```python
from build123d import *

# Parameters (mm, degrees)
BOSS_EXTRUDE1_DEPTH = 1.524


with BuildPart() as part:
    # Sketch1 → Boss-Extrude1 (new body)
    with BuildSketch(Plane.XY):
        with BuildLine():
            Line((70.351759676, -1.540442282), (70.351759676, 0))
            Line((70.351759676, 0), (64.929759758, 0))
            ThreePointArc((64.929759758, 0), (64.792973258, 0.011875), (64.660279583, 0.047144684))
            ThreePointArc((64.660279583, 0.047144684), (62.28963908, 2.412826115), (62.588919113, 5.748514423))
            ThreePointArc((62.588919113, 5.748514423), (62.67763825, 5.871916038), (62.788250891, 5.976146011))
            ThreePointArc((62.788250891, 5.976146011), (63.205809067, 6.291372891), (63.63152168, 6.595497187))
            Line((63.63152168, 6.595497187), (65.410554861, 4.41654898))
            Line((65.410554861, 4.41654898), (66.591058918, 5.380388267))
            Line((66.591058918, 5.380388267), (64.92449722, 7.421582138))
            ThreePointArc((64.92449722, 7.421582138), (67.556403706, 8.712737588), (70.349637054, 9.602603653))
            Line((70.349637054, 9.602603653), (70.349637054, 5.958967549))
            Line((70.349637054, 5.958967549), (71.873637054, 5.958967549))
            Line((71.873637054, 5.958967549), (71.873637054, 7.844356511))
            ThreePointArc((71.873637054, 7.844356511), (72.72464753, 6.890883011), (73.797539642, 6.196452982))
            ThreePointArc((73.797539642, 6.196452982), (77.23855889, 3.495988283), (80.283555852, 0.355746802))
            ThreePointArc((80.283555852, 0.355746802), (80.451041219, 0.021581778), (80.447017019, -0.35218475))
            ThreePointArc((80.447017019, -0.35218475), (80.395843158, -0.762), (80.447017019, -1.17181525))
            ThreePointArc((80.447017019, -1.17181525), (80.451041219, -1.545581778), (80.283555852, -1.879746802))
            ThreePointArc((80.283555852, -1.879746802), (77.23855889, -5.019988283), (73.797539642, -7.720452982))
            ThreePointArc((73.797539642, -7.720452982), (72.72464753, -8.414883011), (71.873637054, -9.368356511))
            Line((71.873637054, -9.368356511), (71.873637054, -7.482967549))
            Line((71.873637054, -7.482967549), (70.349637054, -7.482967549))
            Line((70.349637054, -7.482967549), (70.349637054, -11.126603653))
            ThreePointArc((70.349637054, -11.126603653), (67.556403706, -10.236737588), (64.92449722, -8.945582138))
            Line((64.92449722, -8.945582138), (66.591058918, -6.904388267))
            Line((66.591058918, -6.904388267), (65.410554861, -5.94054898))
            Line((65.410554861, -5.94054898), (63.63152168, -8.119497187))
            ThreePointArc((63.63152168, -8.119497187), (63.205809068, -7.815372891), (62.788250891, -7.500146011))
            ThreePointArc((62.788250891, -7.500146011), (62.67763825, -7.395916038), (62.588919113, -7.272514424))
            ThreePointArc((62.588919113, -7.272514424), (62.262802552, -4.01311856), (64.509301597, -1.629160622))
            ThreePointArc((64.509301597, -1.629160622), (64.654260243, -1.585608721), (64.804850415, -1.570364804))
            Line((64.804850415, -1.570364804), (70.351759676, -1.540442282))
        make_face()
    extrude(amount=BOSS_EXTRUDE1_DEPTH)


solid = part.part
```
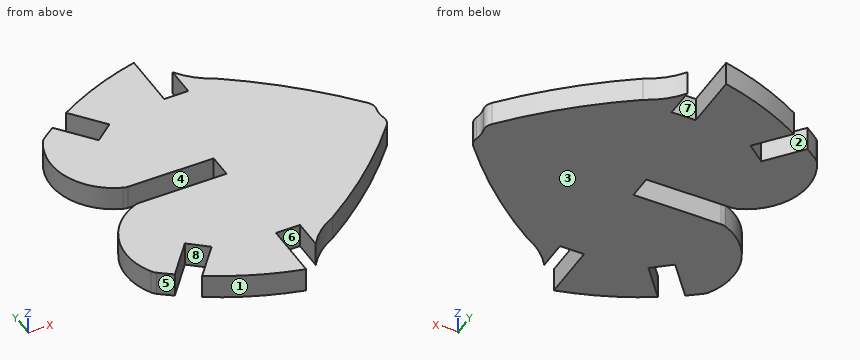
Verification items for the finished model (mm, model axes). Face numbers are marked on the shaded views. A direction names the side the tool comes from. Round coordinates to 2 decimals unless told otherwise and drop trailing zeros. Order: outer loops, then holes, each group sorted by start corner. A loop starts at its lowest first (then second) coordinate and runs counter-clockwise, first axis right, second up. Notation, with made-up numbers: (49, 74) -> (85, 74) arc R20 ccw to (85, 81) -> close; hole circle Ø5 at (29.5, 86). An arc over 180 degrees is marked (long way). Put each result on its own line as item: value. Start each with the question number.
(1) Depth check by flat-ended pin: pin 1 Ø0.5 at (x, z) = (66.5, 1) entering from -Y; pin 2 Ø0.5 at (y, z) = (8, 1) entering from +X; pin 3 Ø0.5 at (y, z) = (-8.5, 0.5) entering from -X; pin 4 Ø8 at (x, y) = (77, 5) entering from -Z. Enter the tip coordinate at first touch or a pass-through.
(2) Section check D-D (y = -2.5). Enter the section's corners in (x, z) (3 decimals), then the cut area to 3 significant figures.
(3) Draft check along Y on the marked faces 1, 2 and 3. Enter one of: +Y half, -Y half, draft (parallel to the pull), parting line (faces both ways), or undercut.
(4) Material ranges on line 1 along Y through (x, z) = (66.5, 1); line 2 along X through (y, z) = (-9, 0.8); line 3 along Y through (x, z) = (67.5, 1.4), recorded low to high.
(5) Section check B-B (y = 7). Enter the section's corners in (x, z), then the cut area to 3 significant figures.
(6) Tool access check on the marked faces 4, 5, 6, 7 and 8. Record the directions out of +Z, -Z, +X, -X, +Y, -Y that give a thin tool (end or side, any length) a straight path to the whole face; none if there is none.
(7) Section check A-A (x = 69.25). Enter the section's corners in (y, z).
Completed:
1. pin 1: stops at y = -9.89
1. pin 2: stops at x = 71.94
1. pin 3: stops at x = 65.08
1. pin 4: stops at z = 0
2. outline: (63.202, 0) -> (79.745, 0) -> (79.745, 1.524) -> (63.202, 1.524) -> close
2. area: 25.2 mm2
3. face 1: -Y half
3. face 2: undercut
3. face 3: draft
4. line 1: y = -9.78 to -7.02, -6.83 to -1.56, 0 to 5.31, 5.49 to 8.25
4. line 2: x = 65.02 to 70.35, 71.87 to 72.15
4. line 3: y = -10.21 to -1.56, 0 to 8.69
5. outline: (65.27, 0) -> (70.35, 0) -> (70.35, 1.52) -> (65.27, 1.52) -> close; (71.87, 0) -> (72.6, 0) -> (72.6, 1.52) -> (71.87, 1.52) -> close
5. area: 8.85 mm2
6. face 4: +Z, -Z, -X
6. face 5: +Z, -Z, -X, -Y
6. face 6: +Z, -Z, -Y
6. face 7: +Z, -Z, +Y
6. face 8: +Z, -Z
7. outline: (-10.83, 0) -> (-1.55, 0) -> (-1.55, 1.52) -> (-10.83, 1.52) -> close; (0, 0) -> (9.31, 0) -> (9.31, 1.52) -> (0, 1.52) -> close
